Job drawing, mm, ordinate dimensions from the low corner. One solid piece. A direction names the side the tool comes from. Round coordinates to 2 decimals unless told otherwise and drop trailing zeros. Order: outer loops, then holes, each group sorted by start corner. A loop starts at its lowest first (then second) coordinate and runs counter-clockwise, first axis right, second up. Notation, with made-up numbers: M 59,51.25 L 94,51.25 A15 ccw 94,55.25 Z; hole C 88,-36.5 d3. An arc over 180 degrees is marked long. Answer as a JSON object with one key per item and string values. Group by question number.
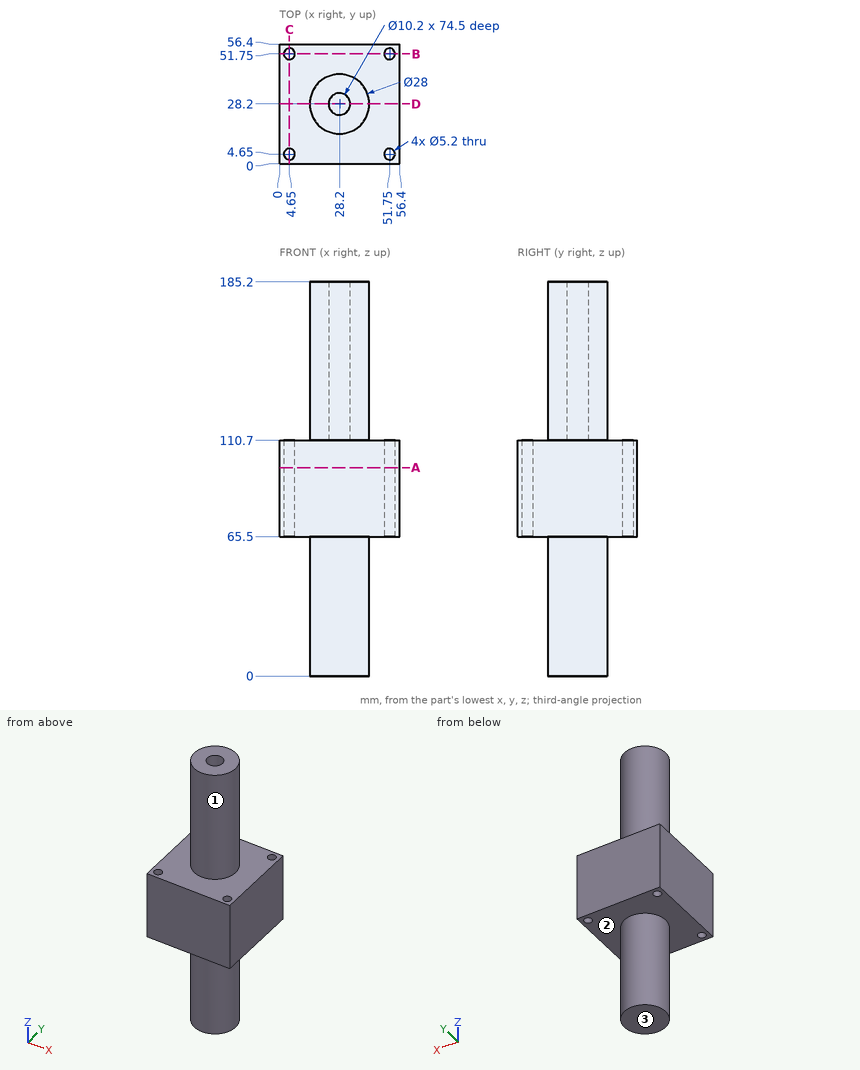
Item 1: Cut at D-D, the plane y = 28.2. Give the cut face in (x, z), and give its area (3 significant figures).
Item 2: 3-axis set-ups, long thin cutter, end or side, ignore diameter. For the marked faces 1, 2 and 3: which of +Z, -Z, +X, -X, +Y, -Y reach the whole face in a straight line?
Item 3: Drill centre lines: line 1 (Y direction, x = 51.75, z = 100); line 2 (X direction, y = 5, z = 88.5); line 3 (Y direction, x = 28.2, z = 153). Where is each one in solid material? Low to high. Write a range as [from, to].
Item 4: Flat gauge pins, fed straight in: pin 1 Ø2 at (x, y) = (32.5, 13.5) entering from -Z; pin 2 Ø5 at (x, y) = (28, 29.5) entering from +Z; pin 3 Ø17 at (x, y) = (39.5, 31.5) entering from -Z; pin 4 Ø8 at (y, z) = (40.5, 30) entering from -X. Where does each tip first touch, or does it go through?
Item 5: Cut at A-A, the plane z = 98. Give the cut face in (x, y), and give its area (3 significant figures).
Item 6: Cut at B-B, the plane y = 51.75. Give the cut face in (x, z), and give its area (3 significant figures).
Response values:
{
 "1": {"outline": "M 0,65.5 L 14.2,65.5 L 14.2,0 L 42.2,0 L 42.2,65.5 L 56.4,65.5 L 56.4,110.7 L 42.2,110.7 L 42.2,185.2 L 33.3,185.2 L 33.3,110.7 L 23.1,110.7 L 23.1,185.2 L 14.2,185.2 L 14.2,110.7 L 0,110.7 Z", "area": "5,710 mm^2"},
 "2": {"face 1": "+Z", "face 2": "-Z", "face 3": "-Z, +X, -X, +Y, -Y"},
 "3": {"line 1": "[0, 2.05], [7.25, 49.15], [54.35, 56.4]", "line 2": "[0, 2.07], [7.23, 49.17], [54.33, 56.4]", "line 3": "[14.2, 23.1], [33.3, 42.2]"},
 "4": {"pin 1": "z = 65.5", "pin 2": "z = 110.7", "pin 3": "z = 0", "pin 4": "x = 16.93"},
 "5": {"outline": "M 0,0 L 56.4,0 L 56.4,56.4 L 0,56.4 Z; hole C 4.65,4.65 d5.2; hole C 4.65,51.75 d5.2; hole C 51.75,4.65 d5.2; hole C 51.75,51.75 d5.2", "area": "3,100 mm^2"},
 "6": {"outline": "M 0,65.5 L 2.05,65.5 L 2.05,110.7 L 0,110.7 Z; M 7.25,65.5 L 49.15,65.5 L 49.15,110.7 L 7.25,110.7 Z; M 54.35,65.5 L 56.4,65.5 L 56.4,110.7 L 54.35,110.7 Z", "area": "2,080 mm^2"}
}
